```python
from build123d import *

# Parameters (mm, degrees)
SKETCH2_W           = 25.4
SKETCH2_H           = 25.4
BOSS_EXTRUDE1_DEPTH = 127
SKETCH4_W           = 19.05
SKETCH4_H           = 19.05
CUT_EXTRUDE1_DEPTH  = 129.263712717
SKETCH5_R           = 3.2639
CUT_EXTRUDE2_DEPTH  = 304.8
SKETCH6_R           = 3.2639
CUT_EXTRUDE3_DEPTH  = 131.136274728
SKETCH7_R           = 3.2639
CUT_EXTRUDE4_DEPTH  = 131.136274728


with BuildPart() as part:
    # Sketch2 → Boss-Extrude1 (new body)
    with BuildSketch(Plane.XY):
        Rectangle(SKETCH2_W, SKETCH2_H)
    extrude(amount=BOSS_EXTRUDE1_DEPTH)

    # Sketch4 → Cut-Extrude1 (cut, through all)
    with BuildSketch(Plane.XY):
        Rectangle(SKETCH4_W, SKETCH4_H)
    extrude(amount=CUT_EXTRUDE1_DEPTH, mode=Mode.SUBTRACT)

    # Sketch5 → Cut-Extrude2 (cut)
    with BuildSketch(Plane(origin=(0, 12.7, 0), x_dir=(1, 0, 0), z_dir=(0, 1, 0))):
        with Locations(Location((0, -25.4, 0), (0, 0, 270))):
            Circle(SKETCH5_R)
    extrude(amount=-CUT_EXTRUDE2_DEPTH, mode=Mode.SUBTRACT)

    # Sketch6 → Cut-Extrude3 (cut, through all)
    with BuildSketch(Plane(origin=(0, 12.7, 0), x_dir=(1, 0, 0), z_dir=(0, 1, 0))):
        with Locations(Location((0, -76.2, 0), (0, 0, 270))):
            Circle(SKETCH6_R)
    extrude(amount=-CUT_EXTRUDE3_DEPTH, mode=Mode.SUBTRACT)

    # Sketch7 → Cut-Extrude4 (cut, through all)
    with BuildSketch(Plane.ZY.offset(12.7)):
        with Locations((38.1, 0)):
            Circle(SKETCH7_R)
        with Locations((112.776, 0)):
            Circle(SKETCH7_R)
    extrude(amount=-CUT_EXTRUDE4_DEPTH, mode=Mode.SUBTRACT)


solid = part.part
```
Build history of the part. All positions in model axes, mm. A direction names the side the tool comes from. Coordinates: 2 decimals unless noted, no trailing zeros. Order: outer loops, then holes, each group sorted by start corner. A loop starts at its lowest first (then second) coordinate and runs counter-clockwise, first axis right, second up. Notation, with made-up numbers: M 41,64.5 L 85,64.5 A33 cw 85,102.5 Z; hole C 34,66.25 d5. An arc over 180 degrees is marked long. One line per question, with ' | ' between items. Start each with the question number.
1. Cut at B-B (y = 0). Write the cut outline in (x, z) (3 decimals), plus the area to 3 significant figures.
2. Mould opens along Y. For faces 3 (the face through (0, 12.7, 63)), 4 (the face through (0, -12.7, 63)), 5 (the face through (-1.25, 11.135, 28.415)), 6 (the face through (0, -9.525, 63)) say: +Y half, -Y half, draft (parallel to the pull), parting line (faces both ways), or undercut.
3. Tool access for faces 1 (the face through (-9.525, 0, 63)), 2 (the face through (12.7, 0, 63)): list every direction of +Z, -Z, +X, -X, +Y, -Y with a clear straight run to the whole face (end or side of a thin tool).
4. Wall check: line 1 along X through (y, z) = (0.5, 79.5) (3 decimals); line 2 along Z through (x, y) = (-1, -11.5). Give the ranges that are in metal, low to high. Write a range as [from, to].
5. Cut at D-D (x = -2). Write the cut outline in (y, z) (3 decimals).
6. Cut at C-C (y = -6.5). Write the cut outline in (x, z) (3 decimals), plus the area to 3 significant figures.
7. Cut at A-A (z = 76.2). Write the cut outline in (x, y) (3 decimals), plus the area to 3 significant figures.
The answers:
1) outline: M -12.7,0 L -9.525,0 L -9.525,34.836 L -12.7,34.836 Z; M -12.7,41.364 L -9.525,41.364 L -9.525,109.512 L -12.7,109.512 Z; M -12.7,116.04 L -9.525,116.04 L -9.525,127 L -12.7,127 Z; M 9.525,0 L 12.7,0 L 12.7,34.836 L 9.525,34.836 Z; M 9.525,41.364 L 12.7,41.364 L 12.7,109.512 L 9.525,109.512 Z; M 9.525,116.04 L 12.7,116.04 L 12.7,127 L 9.525,127 Z | area: 724 mm2
2) face 3: +Y half | face 4: -Y half | face 5: draft | face 6: undercut
3) face 1: +Z, -Z | face 2: +Z, -Z, +X, +Y, -Y
4) line 1: x = [-12.7, -9.525], [9.525, 12.7] | line 2: z = [0, 22.29], [28.51, 73.09], [79.31, 127]
5) outline: M -12.7,0 L -9.525,0 L -9.525,22.821 L -12.7,22.821 Z; M -12.7,27.979 L -9.525,27.979 L -9.525,73.621 L -12.7,73.621 Z; M -12.7,78.779 L -9.525,78.779 L -9.525,127 L -12.7,127 Z; M 9.525,0 L 12.7,0 L 12.7,22.821 L 9.525,22.821 Z; M 9.525,27.979 L 12.7,27.979 L 12.7,73.621 L 9.525,73.621 Z; M 9.525,78.779 L 12.7,78.779 L 12.7,127 L 9.525,127 Z
6) outline: M -12.7,0 L -9.525,0 L -9.525,127 L -12.7,127 Z; M 9.525,0 L 12.7,0 L 12.7,127 L 9.525,127 Z | area: 806 mm2
7) outline: M -12.7,-12.7 L -3.264,-12.7 L -3.264,-9.525 L -9.525,-9.525 L -9.525,9.525 L -3.264,9.525 L -3.264,12.7 L -12.7,12.7 Z; M 3.264,-12.7 L 12.7,-12.7 L 12.7,12.7 L 3.264,12.7 L 3.264,9.525 L 9.525,9.525 L 9.525,-9.525 L 3.264,-9.525 Z | area: 241 mm2
